For this review, take the finished solid that the model builds, in its own axes (mm). A direction names the side the tool comes from. Coordinates: 2 decimals unless noted, no trailing zeros. Order: outer loops, then holes, each group sorted by start corner. A loop starts at its lowest first (then second) coordinate and runs counter-clockwise, first axis right, second up. Notation, with made-up numbers: (37, -19) -> (86, -19) arc R33 cw to (86, 9) -> close; hole circle Ø9 at (-39.75, 30). An arc over 180 degrees is marked (long way). Answer as a JSON object with one key per item and string values. Group by question number.
1) Machinability: for faces 4 (the flat face through (0, 1, 17)), 5 (the cylindrical face through (1.457, 0.822, 30.578)), which of the approach directions +Z, -Z, +X, -X, +Y, -Y give a long, thin tool a straight path to every point of the face, cutting with its end or side? Answer none if there is none.
2) Add section B-B, the plane y = 2.25. Write out the cut boundary in (x, z), then the cut area to 3 significant figures.
3) Draft analysis for pull direction Y (two halves, no side actions). For faces 1 (the flat face through (1, 2.85, 17)), 2 (the flat face through (2.7, -2, 17)), 3 (the cylindrical face through (0.5, -2.46, 5.04)), state which applies: +Y half, -Y half, draft (parallel to the pull), parting line (faces both ways), or undercut.
4) For pin 1 (2 mm diameter, centred on x = -0.5, y = 1.5, fed in from -Z); pin 2 (1.4 mm diameter, centred on y = 1, z = 10.5, fed in from -X); pin 3 (0.6 mm diameter, centred on x = -1, z = 23.5, fed in from +Y), all flat-tipped, find the tip position at first contact; note any pin that passes through.
5) Wall thickness on L1, parallel to Z at x = -0.8, y = -2; L2, parallel to Z at x = 2.35, y = -2.25; L3, parallel to Y at x = -0.15, z = 29: over which ranges is each line inside the solid? List them lowest first.
6) Add section C-C, the plane z = 3.5. Write out the cut boundary in (x, y), then the cut area to 3 significant figures.
7) Add section A-A, the plane z = 26.5. Write out the cut boundary in (x, y), then the cut area to 3 significant figures.
8) Add section D-D, the plane x = -0.35. Count the separate pieces of the cut face and the enclosed holes in it, then the cut area to 3 significant figures.
from build123d import *

# Parameters (mm, degrees)
F1_DEPTH = 35
F3_R     = 0.895736
F3_R_2   = 0.920741
F4_DEPTH = 6.743983
F5_R     = 1.925
F6_DEPTH = 2.75


with BuildPart() as f1:
    # F0 (on Top) → F1 (new body)
    with BuildSketch(Plane.XY):
        Polygon((0, 2.85), (0, 0), (-1.2, 0), (-1.2, -6.15), (2.7, -6.15), (2.7, 2.85), align=None)
    extrude(amount=F1_DEPTH)

    # F3 (on face) → F4 (cut, through all)
    with BuildSketch(Plane(origin=(3.300132, 1.20115, 0), x_dir=(-0.34202, 0.939693, 0), z_dir=(0.939693, 0.34202, 0))):
        with Locations((-1.561705, 30)):
            Circle(F3_R)
        with Locations((-1.561705, 5)):
            Circle(F3_R_2)
    extrude(amount=-F4_DEPTH, mode=Mode.SUBTRACT)

    # F5 (on face) → F6 (cut)
    with BuildSketch(Plane(origin=(3.300132, 1.20115, 0), x_dir=(-0.34202, 0.939693, 0), z_dir=(0.939693, 0.34202, 0))):
        with Locations((-1.561705, 30)):
            Circle(F5_R)
        with Locations((-1.561705, 5)):
            Circle(F5_R)
    extrude(amount=-F6_DEPTH, mode=Mode.SUBTRACT)


solid = f1.part
Output values:
{
 "1": {"face 4": "+Z, -Z, -X, +Y", "face 5": "none"},
 "2": {"outline": "(0, 0) -> (2.7, 0) -> (2.7, 35) -> (0, 35) -> close", "area": "94.5 mm²"},
 "3": {"face 1": "+Y half", "face 2": "draft", "face 3": "undercut"},
 "4": {"pin 1": "stops at z = 0", "pin 2": "stops at x = 0", "pin 3": "stops at y = 0"},
 "5": {"L1": "z = 0 to 4.08, 5.92 to 29.11, 30.89 to 35", "L2": "z = 0 to 3.63, 6.37 to 28.63, 31.37 to 35", "L3": "y = -6.15 to 0"},
 "6": {"outline": "(-1.2, -6.15) -> (2.7, -6.15) -> (2.7, -1.96) -> (1.66, -2.34) -> (0.84, -0.07) -> (2.7, 0.6) -> (2.7, 2.85) -> (0, 2.85) -> (0, 0) -> (-1.2, 0) -> close", "area": "28.0 mm²"},
 "7": {"outline": "(-1.2, -6.15) -> (2.7, -6.15) -> (2.7, 2.85) -> (0, 2.85) -> (0, 0) -> (-1.2, 0) -> close", "area": "31.7 mm²"},
 "8": {"separate pieces": "1", "enclosed holes": "2", "area": "210 mm²"}
}
